from build123d import *

# Parameters (mm, degrees)
F2_R = 2


with BuildPart() as f1:
    # F0 (on Front) → F1 (revolve)
    with BuildSketch(Plane.XZ):
        Polygon((38, 0), (0, 0), (0, -3), (12.181578204, -3), (14, -3), (14, -35), (-6, -35), (-6, -41), (44, -41), (44, -35), (24, -35), (24, -3), (38, -3), align=None)
    revolve(axis=Axis((16.9901512563, 0, -53), (1, 0, 0)))

    # F2
    f2_edges = [f1.edges().sort_by_distance(p)[0] for p in [
        (14, 0, -103),
        (24, 0, -103),
    ]]
    fillet(f2_edges, radius=F2_R)


solid = f1.part
Work out the finished part from the listing and answer in its coordinate system (mm). A direction names the side the tool comes from. Coordinates: 2 decimals unless noted, no trailing zeros. Write each loop counter-clockwise with the first axis right and the second up, starting at its lowest first coordinate (ties: lowest second). Pieces come first, ordered by that corner, then holes. Notation, with made-up numbers: M 27.25,29.5 L 62.25,29.5 A27 ccw 62.25,60.5 Z; hole C 62,34.5 d5. An arc over 180 degrees is marked long. Use one line per item in the form item = value. Start each with the question number.
1. The part is cut by section A-A (z = -53). Give the vertices of the cut face in (x, y), plus the area to 3 significant figures.
2. The mould has two halves that part along Y. Classify faces 4 (the face through (0, -32, -14)), 5 (the face through (18.734, -15.92, -2.447)), 6 (the face through (33.86, -5.407, -35.831)): released by +Y, released by -Y, zero draft, split by the parting line, or undercut.
3. Straight lines are drawn through the part: probe 1 along Z at (x, y) = (31, 0); probe 2 along Y at (x, z) = (32, -53); probe 3 along Z at (x, y) = (10.5, 9.5). For each, find the intervals that lie inside material, in ascending order. Write a range as from..to.
4. A tool of negligible diameter and unlimited length cuts with its end or side. For faces 1 (the face through (32, 30, -93)), 2 (the face through (14, 21, -54)), 3 (the face through (44, 4, -65)), from which of +Z, -Z, +X, -X, +Y, -Y can it reach the whole face along a straight path? Write none if from no direction.
5. Each of these flat-tipped pins is pushed along its axis until it touches: P1, Ø1.5, axis at y = 40, z = -82, coming from the -X side; P2, Ø1.5, axis at x = 14, y = 41.5, coming from the -Z side; P3, Ø1.5, axis at x = 0.5, z = -23, coming from the +Y side; P4, Ø3, axis at y = 10.5, z = -37, coming from the -X side. Where does it stop, or does it pass through?
6. The part is cut by section B-B (y = 0). Give the vertices of the cut face in (x, z).
Evaluation:
q1.outline = M -6,-18 L 14,-18 L 14,-48 A2 cw 12,-50 L 0,-50 L 0,-53 L 38,-53 L 38,-50 L 26,-50 A2 cw 24,-48 L 24,-18 L 44,-18 L 44,-12 L -6,-12 Z; M -6,12 L 44,12 L 44,18 L 24,18 L 24,48 A2 cw 26,50 L 38,50 L 38,53 L 0,53 L 0,50 L 12,50 A2 cw 14,48 L 14,18 L -6,18 Z
q1.area = 1,470 mm^2
q2.face_4 = zero draft
q2.face_5 = split by the parting line
q2.face_6 = undercut
q3.probe_1 = -106..-103, -71..-65, -41..-35, -3..0
q3.probe_2 = -53..-50, -18..-12, 12..18, 50..53
q3.probe_3 = -105.14..-102.09, -68.29..-60.33, -45.67..-37.71, -3.91..-0.86
q4.face_1 = +X
q4.face_2 = -X
q4.face_3 = +Z, -Z, +X, +Y, -Y
q5.P1 = 0
q5.P2 = -86.89
q5.P3 = 44.2
q5.P4 = -6
q6.outline = M -6,-71 L 14,-71 L 14,-101 A2 cw 12,-103 L 0,-103 L 0,-106 L 38,-106 L 38,-103 L 26,-103 A2 cw 24,-101 L 24,-71 L 44,-71 L 44,-65 L -6,-65 Z; M -6,-41 L 44,-41 L 44,-35 L 24,-35 L 24,-5 A2 cw 26,-3 L 38,-3 L 38,0 L 0,0 L 0,-3 L 12,-3 A2 cw 14,-5 L 14,-35 L -6,-35 Z
